For this review, take the finished solid that the model builds, in its own axes (mm). Give positions to 0.01 mm unless a question says otherwise; leave off trailing zeros. Write each loop counter-clockwise with the first axis right and the second up, starting at its lowest first coordinate (ties: lowest second). Pieces come first, ordered by that corner, then holes.
Autodesk Inventor part; units mm, degrees
ref_plane "YZ Plane" through (0, 0, 0) normal (1, 0, 0) x (0, 1, 0)
ref_plane "XZ Plane" through (0, 0, 0) normal (0, 1, 0) x (-1, 0, 0)
ref_plane "XY Plane" through (0, 0, 0) normal (0, 0, 1) x (1, 0, 0)
sketch "Sketch1" plane through (0, 0, 0) normal (0, 0, 1) x (1, 0, 0)
  circle A0 centre (0, 0) radius 3.5
  dimension "d0" = 7
extrude "Extrusion1" add sketch "Sketch1" along normal blind 1.5
sketch "Sketch2" plane through (0, 0, 1.5) normal (0, 0, 1) x (1, 0, 0)
  circle A0 centre (0, 0) radius 2.5
  dimension "d3" = 5
extrude "Extrusion2" add sketch "Sketch2" along normal blind 5
sketch "Sketch3" plane through (0, 0, 0) normal (0, 0, -1) x (-1, 0, 0)
  circle A0 centre (0, 0) radius 3.5
hole "Hole1" at (0, 0, 0) direction (0, 0, 1) diameter 2.459 end through all
sketch "Sketch4" plane through (0, 0, 0) normal (0, 0, -1) x (-1, 0, 0)
  line L0 (-0.35, 3.9217) -> (0.35, 3.9217)
  line L1 (0.35, 3.9217) -> (0.35, -3.9092)
  line L2 (0.35, -3.9092) -> (-0.35, -3.9092)
  line L3 (-0.35, -3.9092) -> (-0.35, 3.9217)
  point P0 (0, 0)
  dimension "d13" = 0.7
  dimension "d14" = 0.35
extrude "Extrusion3" cut sketch "Sketch4" against normal blind 0.7
thread "Thread1"
properties part number "screw-mount"
(1) For L1, parallel to Y at x = 0, z = 3.5; L2, parallel to X at y = 0, z = 1; L3, parallel to Z at x = 3.25, y = 0, list the stretches that pass through material, from the lowest coordinate up.
(2) We need section A-A (y = 0). Write out the cut boundary in (x, z), and give its area (3 significant figures).
(3) The part is to be moulded in two halves that separate along Z. For faces 1 (the flat face through (2, -2, 1.5)), 2 (the cylindrical face through (-0.54, 2.44, 3.96)), 3 (the flat face through (2, 0, 0)), say which applies: +Z half, -Z half, draft (parallel to the pull), parting line (faces both ways), or undercut.
(4) We need section D-D (z = 2.25). Write out the cut boundary in (x, y).
(5) We need section C-C (z = 0.5). Write out the cut boundary in (x, y).
(6) We need section B-B (x = 0). Write out the cut boundary in (y, z).
(7) Clearance check with flat-ended pins moving along their axes: pin 1 Ø3 at (x, z) = (-0.5, 5) entering from -Y; pin 2 Ø0.6 at (y, z) = (-2, 0.5) entering from -X; pin 3 Ø1 at (x, z) = (0, 2.5) entering from +Y. State where each tip first meets the part, or that it passes through.
The answers:
1. L1: y = -2.5 to -1.23, 1.23 to 2.5
1. L2: x = -3.5 to -1.23, 1.23 to 3.5
1. L3: z = 0 to 1.5
2. outline: (-3.5, 0) - (-1.23, 0) - (-1.23, 6.5) - (-2.5, 6.5) - (-2.5, 1.5) - (-3.5, 1.5) - close; (1.23, 0) - (3.5, 0) - (3.5, 1.5) - (2.5, 1.5) - (2.5, 6.5) - (1.23, 6.5) - close
2. area: 19.5 mm2
3. face 1: +Z half
3. face 2: draft
3. face 3: -Z half
4. outline: circle Ø5 at (0, 0); hole circle Ø2.46 at (0, 0)
5. outline: (-0.35, -3.48) - (-0.35, -1.18) arc R1.23 cw to (-0.35, 1.18) - (-0.35, 3.48) arc R3.5 ccw to start; (0.35, -3.48) arc R3.5 ccw to (0.35, 3.48) - (0.35, 1.18) arc R1.23 cw to (0.35, -1.18) - close
6. outline: (-3.5, 0.7) - (-1.23, 0.7) - (-1.23, 6.5) - (-2.5, 6.5) - (-2.5, 1.5) - (-3.5, 1.5) - close; (1.23, 0.7) - (3.5, 0.7) - (3.5, 1.5) - (2.5, 1.5) - (2.5, 6.5) - (1.23, 6.5) - close
7. pin 1: stops at y = -2.5
7. pin 2: stops at x = -3.06
7. pin 3: stops at y = 2.5
